Geometry check sheet. Reference: the model listing, model coordinates, mm. Coordinates: 2 decimals unless noted, no trailing zeros. Loops run counter-clockwise (first coordinate to the right, second up) from the corner with the lowest first, then second, coordinate; pieces in that order, holes last.
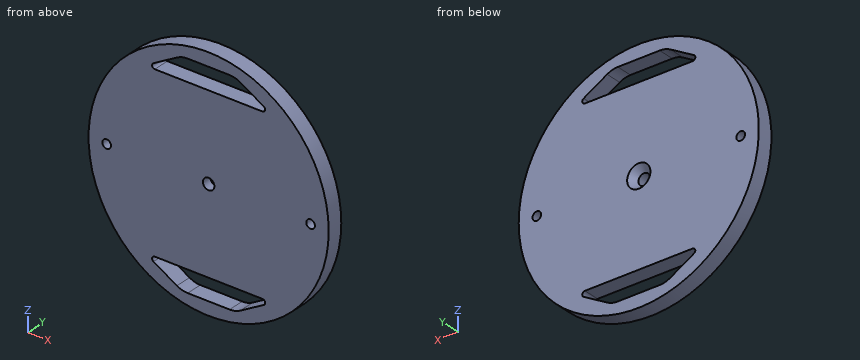
from build123d import *

# Parameters (mm, degrees)
SKETCH2_R                                        = 71.0565
BOSS_EXTRUDE1_DEPTH                              = 9.525
TAP_DRILL_FOR_1_4_20_TAP1_D                      = 5.1054
CSK_FOR_1_4_FLAT_HEAD_MACHINE_SCREW1_D           = 6.7564
CSK_FOR_1_4_FLAT_HEAD_MACHINE_SCREW1_CSINK_D     = 13.7668
CSK_FOR_1_4_FLAT_HEAD_MACHINE_SCREW1_CSINK_ANGLE = 82
CUT_EXTRUDE1_START                               = -10.525
CUT_EXTRUDE1_DEPTH                               = 11.525
FILLET1_R                                        = 12.7
FILLET2_R                                        = 1.5875
FILLET1_OF_MIRROR1_R                             = 12.7
FILLET2_OF_MIRROR1_R                             = 1.5875


with BuildPart() as part:
    # Sketch2 → Boss-Extrude1 (new body)
    with BuildSketch(Plane(origin=(0, 0, 0), x_dir=(1, 0, 0), z_dir=(0, 1, 0))):
        Circle(SKETCH2_R)
    extrude(amount=BOSS_EXTRUDE1_DEPTH)

    # Tap Drill for 1/4-20 Tap1 (through all)
    with Locations(Plane(origin=(0, 9.525, 0), x_dir=(1, 0, 0), z_dir=(0, 1, 0))):
        with Locations((-60.325, 0), (60.325, 0)):
            Hole(TAP_DRILL_FOR_1_4_20_TAP1_D / 2)

    # CSK for 1/4 Flat Head Machine Screw1 (through all)
    with Locations(Plane(origin=(0, 9.525, 0), x_dir=(1, 0, 0), z_dir=(0, 1, 0))):
        with Locations((0, 0)):
            CounterSinkHole(CSK_FOR_1_4_FLAT_HEAD_MACHINE_SCREW1_D / 2, CSK_FOR_1_4_FLAT_HEAD_MACHINE_SCREW1_CSINK_D / 2, counter_sink_angle=CSK_FOR_1_4_FLAT_HEAD_MACHINE_SCREW1_CSINK_ANGLE)

    # Sketch8 → Cut-Extrude1 (cut)
    with BuildSketch(Plane(origin=(0, 9.525, 0), x_dir=(1, 0, 0), z_dir=(0, 1, 0)).offset(CUT_EXTRUDE1_START)):
        Polygon((-37.8, 50.5), (-15.802954744, 63.2), (15.802954744, 63.2), (37.8, 50.5), align=None)
    cut_extrude1 = extrude(amount=CUT_EXTRUDE1_DEPTH, mode=Mode.SUBTRACT)

    # Fillet1
    fillet1_edges = [part.edges().sort_by_distance(p)[0] for p in [
        (-15.802954744, 4.7625, -63.2),
        (15.802954744, 4.7625, -63.2),
    ]]
    fillet(fillet1_edges, radius=FILLET1_R)

    # Fillet2
    fillet2_edges = [part.edges().sort_by_distance(p)[0] for p in [
        (37.8, 4.7625, -50.5),
        (-37.8, 4.7625, -50.5),
    ]]
    fillet(fillet2_edges, radius=FILLET2_R)

    # Mirror1: Cut-Extrude1 across plane
    add(cut_extrude1.mirror(Plane.XY), mode=Mode.SUBTRACT)

    # Fillet1 of Mirror1
    fillet1_of_mirror1_edges = [part.edges().sort_by_distance(p)[0] for p in [
        (-15.802954744, 4.7625, 63.2),
        (15.802954744, 4.7625, 63.2),
    ]]
    fillet(fillet1_of_mirror1_edges, radius=FILLET1_OF_MIRROR1_R)

    # Fillet2 of Mirror1
    fillet2_of_mirror1_edges = [part.edges().sort_by_distance(p)[0] for p in [
        (37.8, 4.7625, 50.5),
        (-37.8, 4.7625, 50.5),
    ]]
    fillet(fillet2_of_mirror1_edges, radius=FILLET2_OF_MIRROR1_R)


solid = part.part
1) Section check D-D on x = -14.5. Record the cut outline in (y, z) (3 decimals), and give its area (3 significant figures).
Data:
outline: (0, -69.561) - (9.525, -69.561) - (9.525, -63.025) - (0, -63.025) - close; (0, -50.5) - (9.525, -50.5) - (9.525, 50.5) - (0, 50.5) - close; (0, 63.025) - (9.525, 63.025) - (9.525, 69.561) - (0, 69.561) - close
area: 1,090 mm2
2) Section check B-B on z = 0. Record the cut outline in (x, y) (1 decimal).
Data:
outline: (-71.1, 0) - (-62.9, 0) - (-62.9, 9.5) - (-71.1, 9.5) - close; (-57.8, 0) - (-3.4, 0) - (-3.4, 5.5) - (-6.9, 9.5) - (-57.8, 9.5) - close; (3.4, 0) - (57.8, 0) - (57.8, 9.5) - (6.9, 9.5) - (3.4, 5.5) - close; (62.9, 0) - (71.1, 0) - (71.1, 9.5) - (62.9, 9.5) - close
3) Section check C-C on y = 7. Count the separate pieces of the cut face and the enclosed holes in it, and give its area (3 significant figures).
Data:
separate pieces: 1
enclosed holes: 5
area: 14,400 mm2
4) Section check A-A on x = 0. Record the cut outline in (y, z) (1 decimal).
Data:
outline: (0, -71.1) - (9.5, -71.1) - (9.5, -63.2) - (0, -63.2) - close; (0, -50.5) - (9.5, -50.5) - (9.5, -6.9) - (5.5, -3.4) - (0, -3.4) - close; (0, 3.4) - (5.5, 3.4) - (9.5, 6.9) - (9.5, 50.5) - (0, 50.5) - close; (0, 63.2) - (9.5, 63.2) - (9.5, 71.1) - (0, 71.1) - close
5) Depth check by flat-ended pin: pin 1 (5 mm diameter, centred on x = -3, y = 4, fed in from -Z); pin 2 (4 mm diameter, centred on y = 4.5, z = -48, fed in from -X); pin 3 (5 mm diameter, centred on y = 2.5, z = -27, fed in from +X); pin 4 (4 mm diameter, centred on x = -60.325, z = 0, fed in from +Y). Enter the tip coordinate at first touch or a pass-through.
Data:
pin 1: stops at z = -71.05
pin 2: stops at x = -54.16
pin 3: stops at x = 66.7
pin 4: passes through
6) Material ranges on probe 1 along Z at (x, y) = (0, 2.95); probe 2 along Z at (x, y) = (-14, 4.25); probe 3 along Z at (x, y) = (13, 3.25), recorded low to high.
Data:
probe 1: z = -71.06 to -63.2, -50.5 to -3.38, 3.38 to 50.5, 63.2 to 71.06
probe 2: z = -69.66 to -63.1, -50.5 to 50.5, 63.1 to 69.66
probe 3: z = -69.86 to -63.19, -50.5 to 50.5, 63.19 to 69.86
